from build123d import *

# Parameters (mm, degrees)
SKETCH1_W                = 80
SKETCH1_H                = 20
BOSS_EXTRUDE1_DEPTH      = 2.5
BOSS_EXTRUDE1_DEPTH_BACK = 2.5
BOSS_EXTRUDE2_DEPTH      = 3
FILLET1_R                = 1.5
SKETCH3_R                = 1.2
CUT_EXTRUDE1_DEPTH       = 1
CUT_EXTRUDE1_DEPTH_BACK  = 87
BOSS_EXTRUDE3_START      = 2.5
SKETCH4_R                = 8.75
BOSS_EXTRUDE3_DEPTH      = 7.5


with BuildPart() as part:
    # Sketch1 → Boss-Extrude1 (new body, two sides)
    with BuildSketch(Plane(origin=(0, 0, 0), x_dir=(1, 0, 0), z_dir=(0, 1, 0))) as boss_extrude1_sk:
        Rectangle(SKETCH1_W, SKETCH1_H)
    extrude(amount=BOSS_EXTRUDE1_DEPTH)
    extrude(boss_extrude1_sk.sketch, amount=-BOSS_EXTRUDE1_DEPTH_BACK)

    # Sketch2 → Boss-Extrude2 (add)
    with BuildSketch(Plane(origin=(40, 0, 0), x_dir=(0, 0, -1), z_dir=(1, 0, 0))):
        Polygon((-26, 2.5), (26, 2.5), (26, -10.3), (18, -10.3), (18, -2.5), (-18, -2.5), (-18, -10.3), (-26, -10.3), align=None)
    boss_extrude2 = extrude(amount=BOSS_EXTRUDE2_DEPTH)

    # Mirror2: Boss-Extrude2 across plane
    add(boss_extrude2.mirror(Plane(origin=(0, 0, 0), x_dir=(0, 0, 1), z_dir=(1, 0, 0))))

    # Fillet1
    fillet1_edges = [part.edges().sort_by_distance(p)[0] for p in [
        (43, -10.3, 22),
        (43, -10.3, -22),
        (-43, -10.3, -22),
        (-43, -10.3, 22),
    ]]
    fillet(fillet1_edges, radius=FILLET1_R)

    # Sketch3 → Cut-Extrude1 (cut, two sides)
    with BuildSketch(Plane(origin=(43, 0, 0), x_dir=(0, 0, -1), z_dir=(1, 0, 0))) as cut_extrude1_sk:
        with Locations((22, -0.2)):
            Circle(SKETCH3_R)
        with Locations((-22, -0.2)):
            Circle(SKETCH3_R)
        with Locations((-22, -5.6)):
            Circle(SKETCH3_R)
        with Locations((22, -5.6)):
            Circle(SKETCH3_R)
    extrude(amount=CUT_EXTRUDE1_DEPTH, mode=Mode.SUBTRACT)
    extrude(cut_extrude1_sk.sketch, amount=-CUT_EXTRUDE1_DEPTH_BACK, mode=Mode.SUBTRACT)

    # Sketch4 → Boss-Extrude3 (add)
    with BuildSketch(Plane(origin=(0, 0, 0), x_dir=(1, 0, 0), z_dir=(0, 1, 0)).offset(BOSS_EXTRUDE3_START)):
        Circle(SKETCH4_R)
    extrude(amount=BOSS_EXTRUDE3_DEPTH)


solid = part.part
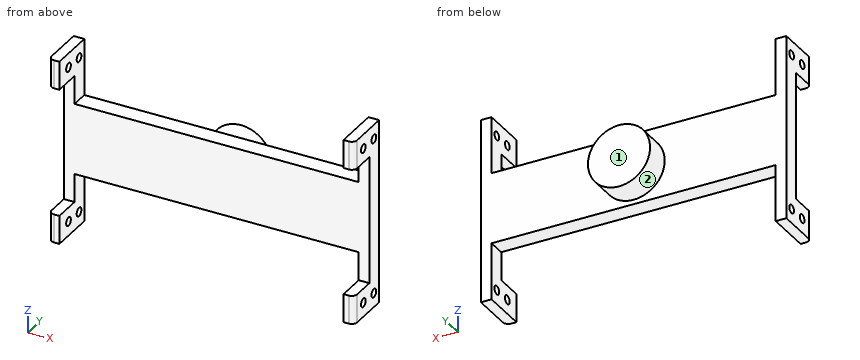
Source: CAD feature listing. Evaluate the final solid. Frame: model axes, mm. Face numbers are marked on the shaded views. A direction names the side the tool comes from. Round coordinates to 2 decimals unless told otherwise and drop trailing zeros. Loops run counter-clockwise (first coordinate to the right, second up) from the corner with the lowest first, then second, coordinate; pieces in that order, holes last. Notation, with made-up numbers: (54, 51.5) -> (61, 51.5) arc R16 ccw to (61, 66.5) -> close; hole circle Ø3 at (7, -4.5). An arc over 180 degrees is marked (long way). Answer as a JSON object with one key per item and string values. Group by question number.
Q1. Section query B-B (y = -0.2). Output: boundary loops of the cut face in (x, z), plus the area to 3 significant figures.
Q2. Section query D-D (x = 0). Output: boundary loops of the cut face in (y, z).
Q3. Section query C-C (z = 22). Output: boundary loops of the cut face in (x, y), plus the area to 3 significant figures.
Q4. Section query A-A (z = -13). Output: boundary loops of the cut face in (x, y).
Q5. Access query for the marked faces 1 and 2. Directions: +Z, -Z, +X, -X, +Y, -Y. A direction counts if a zero-diameter tool reaches every point of the face in a straight line with its end or side. Return the directions, or none.
Q6. Ray query, line 1 (Y direction, x = 41, z = 22); line 2 (X direction, y = -2, z = 18); line 3 (Z direction, x = 17, y = -1.5). Return the intervals inside material, ascending. Write a range as from..to.
Q7. Contact query for flat-ended pins moving along their axis: P1, Ø4, axis at x = 21, z = 6.5, coming from the -Y side; P2, Ø4, axis at y = -4.5, z = -16.5, coming from the -X side; P3, Ø1.5, axis at x = 12.5, y = 0.5, coming from the -Z side; P4, Ø2.5, axis at x = 6.5, y = -1, coming from the +Z side. Output: stop coordinate, or through.
Completed:
{
 "1": {"outline": "(-43, -26) -> (-40, -26) -> (-40, -23.2) -> (-43, -23.2) -> close; (-43, -20.8) -> (-40, -20.8) -> (-40, -10) -> (40, -10) -> (40, -20.8) -> (43, -20.8) -> (43, 20.8) -> (40, 20.8) -> (40, 10) -> (-40, 10) -> (-40, 20.8) -> (-43, 20.8) -> close; (-43, 23.2) -> (-40, 23.2) -> (-40, 26) -> (-43, 26) -> close; (40, -26) -> (43, -26) -> (43, -23.2) -> (40, -23.2) -> close; (40, 23.2) -> (43, 23.2) -> (43, 26) -> (40, 26) -> close", "area": "1,880 mm²"},
 "2": {"outline": "(-2.5, -10) -> (2.5, -10) -> (2.5, -8.75) -> (10, -8.75) -> (10, 8.75) -> (2.5, 8.75) -> (2.5, 10) -> (-2.5, 10) -> close"},
 "3": {"outline": "(-43, -8.8) arc R1.5 ccw to (-41.5, -10.3) -> (-40, -10.3) -> (-40, -6.8) -> (-43, -6.8) -> close; (-43, -4.4) -> (-40, -4.4) -> (-40, -1.4) -> (-43, -1.4) -> close; (-43, 1) -> (-40, 1) -> (-40, 2.5) -> (-43, 2.5) -> close; (40, -10.3) -> (41.5, -10.3) arc R1.5 ccw to (43, -8.8) -> (43, -6.8) -> (40, -6.8) -> close; (40, -4.4) -> (43, -4.4) -> (43, -1.4) -> (40, -1.4) -> close; (40, 1) -> (43, 1) -> (43, 2.5) -> (40, 2.5) -> close", "area": "47.0 mm²"},
 "4": {"outline": "(-43, -2.5) -> (-40, -2.5) -> (-40, 2.5) -> (-43, 2.5) -> close; (40, -2.5) -> (43, -2.5) -> (43, 2.5) -> (40, 2.5) -> close"},
 "5": {"face 1": "+Z, -Z, +X, -X, +Y", "face 2": "+Y"},
 "6": {"line 1": "-10.3..-6.8, -4.4..-1.4, 1..2.5", "line 2": "-43..-40, 40..43", "line 3": "-10..10"},
 "7": {"P1": "y = -2.5", "P2": "x = -43", "P3": "z = -10", "P4": "z = 10"}
}
